The listing builds one solid part. Answer for the finished solid, in the listing's coordinates (mm). A direction names the side the tool comes from. Give positions to 0.01 mm unless a question says otherwise; leave off trailing zeros. Order: outer loops, then holes, each group sorted by start corner. A loop starts at its lowest first (then second) coordinate and runs counter-clockwise, first axis right, second up. Notation, with made-up numbers: (38, 75) - (56, 75) arc R26 ccw to (56, 108) - close; hole circle Ø5 at (-16, 68). An arc over 180 degrees is marked (long way). Use a Markdown table: item, result. Add a question column.
1) Flat-ended cylindrical pins translate along their axes: pin 1 (3 mm diameter, centred on x = 0, y = 4.5, fed in from -Z); pin 2 (1.5 mm diameter, centred on y = 4.5, z = -5, fed in from +X); pin 3 (3 mm diameter, centred on x = -4, y = 2, fed in from -Z). Find the tip coordinate at first contact, or state that the pin passes through.
2) Straight lines are drawn through the part: line 1 (X direction, y = 3.75, z = 0); line 2 (Z direction, x = 0, y = 1.8); line 3 (X direction, y = 4.75, z = -0.5). For each, find the intervals that lie inside material, in ascending order.
3) For faces 1 (the face through (2, 9, 2)), 2 (the face through (10, 2, 4)), 3 (the face through (10, 2, -4)), determine the directions among +Z, -Z, +X, -X, +Y, -Y from which every point of the face is accessible in a straight line to the end or side of a thin tool.
4) Find section A-A, the plane x = 0. Determine the outline of the cut face in (y, z), plus the area to 4 significant figures.
5) Find section C-C, the plane y = 1. Determine the outline of the cut face in (x, z).
6) Find section B-B, the plane z = 0. Determine the outline of the cut face in (x, y), plus the area to 3 significant figures.
7) The mould has two halves that part along X. Classify faces 4 (the face through (11, 5, 0)), 5 (the face through (1.765, 5.056, -4.086)), 6 (the face through (11.905, 2.465, -0.092)), 7 (the face through (18, 2.5, -0.1)): released by +X, released by -X, zero draft, split by the parting line, or undercut.
8) Find section D-D, the plane y = 7.25. Determine the outline of the cut face in (x, z), plus the area to 3 significant figures.
from build123d import *

# Parameters (mm, degrees)
SKETCH_1_R           = 2.1
EXTRUDE_1_DEPTH      = 5
SKETCH_2_R           = 7.5
SKETCH_2_R_2         = 2
EXTRUDE_2_DEPTH      = 4
EXTRUDE_2_DEPTH_BACK = 5
SKETCH_3_R           = 1.85
CUT_EXTRUDE_1_DEPTH  = 12


with BuildPart() as part:
    # 草图1 → 凸台-拉伸1 (new body)
    with BuildSketch(Plane(origin=(0, 0, 0), x_dir=(1, 0, 0), z_dir=(0, 1, 0))):
        with BuildLine():
            Line((0, 4), (14.003, 4))
            ThreePointArc((14.003, 4), (18.003, 0), (14.003, -4))
            Line((14.003, -4), (0, -4))
            ThreePointArc((0, -4), (-4, 0), (0, 4))
        make_face()
        Circle(SKETCH_1_R, mode=Mode.SUBTRACT)
        with Locations((14.003, 0)):
            Circle(SKETCH_1_R, mode=Mode.SUBTRACT)
    extrude(amount=EXTRUDE_1_DEPTH)

    # 草图2 → 凸台-拉伸2 (add, two sides)
    with BuildSketch(Plane(origin=(0, 5, 0), x_dir=(1, 0, 0), z_dir=(0, 1, 0))) as extrude_2_sk:
        Circle(SKETCH_2_R)
        Circle(SKETCH_2_R_2, mode=Mode.SUBTRACT)
    extrude(amount=EXTRUDE_2_DEPTH)
    extrude(extrude_2_sk.sketch, amount=-EXTRUDE_2_DEPTH_BACK)

    # 草图3 → 切除-拉伸1 (cut)
    with BuildSketch(Plane.XY):
        with Locations((0, 4.5)):
            Circle(SKETCH_3_R)
    extrude(amount=-CUT_EXTRUDE_1_DEPTH, mode=Mode.SUBTRACT)


solid = part.part
The answers:
| question | item | result |
|---|---|---|
| 1 | pin 1 | z = 1.32 |
| 1 | pin 2 | x = 6.18 |
| 1 | pin 3 | z = -7.07 |
| 2 | line 1 | -7.5 to -2, 2 to 11.9, 16.1 to 18 |
| 2 | line 2 | -7.5 to -2, 2 to 7.5 |
| 2 | line 3 | -7.48 to -1.94, 1.94 to 11.96, 16.04 to 17.97 |
| 3 | face 1 | +Z, -Z, +X, -X, +Y |
| 3 | face 2 | +Z, +X, +Y, -Y |
| 3 | face 3 | -Z, +X, +Y, -Y |
| 4 | outline | (0, -7.5) - (2.65, -7.5) - (2.65, -2) - (0, -2) - close; (0, 2) - (9, 2) - (9, 7.5) - (0, 7.5) - close; (6.35, -7.5) - (9, -7.5) - (9, -2) - (6.35, -2) - close |
| 4 | area | 78.65 mm2 |
| 5 | outline | (6.34, -4) - (14, -4) arc R4 ccw to (14, 4) - (6.34, 4) arc R7.5 ccw (long way) to start; hole circle Ø4 at (0, 0); hole circle Ø4.2 at (14, 0) |
| 6 | outline | (-7.5, 0) - (-2, 0) - (-2, 9) - (-7.5, 9) - close; (2, 0) - (11.9, 0) - (11.9, 5) - (7.5, 5) - (7.5, 9) - (2, 9) - close; (16.1, 0) - (18, 0) - (18, 5) - (16.1, 5) - close |
| 6 | area | 131 mm2 |
| 7 | face 4 | zero draft |
| 7 | face 5 | undercut |
| 7 | face 6 | undercut |
| 7 | face 7 | released by +X |
| 8 | outline | circle Ø15 at (0, 0); hole circle Ø4 at (0, 0) |
| 8 | area | 164 mm2 |
